Input: part model. Units: mm. Frame: model coordinates. Face numbers are marked on the shaded views. A direction names the side the tool comes from. Give positions to 0.01 mm unless a question says otherwise; leave off trailing zeros. Loops run counter-clockwise (first coordinate to the right, second up) from the corner with the lowest first, then second, coordinate; pieces in that order, holes last. Notation, with made-up numbers: (76, 76) -> (88, 76) arc R19 cw to (88, 106) -> close; hole circle Ø3 at (89, 17.25). An arc over 180 degrees is marked (long way). Answer as a JSON object with one key per item and string values.
```python
from build123d import *

# Parameters (mm, degrees)
F1_ANGLE_BACK = 135
F1_ANGLE      = 270
F3_DEPTH      = 29
F4_DEPTH      = 29


with BuildPart() as f1:
    # F0 (on Front) → F1 (revolve)
    with BuildSketch(Plane.XZ, mode=Mode.PRIVATE) as f1_sk:
        Polygon((0, -4), (0, 4), (-35, 4), (-35, 29), (-43, 29), (-43, -29), (-35, -29), (-35, -4), align=None)
    revolve(f1_sk.sketch.rotate(Axis((0, 0, -1.0322406888), (0, 0, 1)), -F1_ANGLE_BACK), axis=Axis((0, 0, -1.0322406888), (0, 0, 1)), revolution_arc=F1_ANGLE)

    # F2 (on Top) → F3 (join, through all)
    with BuildSketch(Plane.XY):
        Polygon((0, 0), (30.405591591, -30.405591591), (33.941125497, -26.8700576851), (7.0710678119, 0), (33.941125497, 26.8700576851), (30.405591591, 30.405591591), align=None)
    extrude(amount=F3_DEPTH)

    # F4 (add, through all): a face of the model
    f4_faces = [f1.faces().sort_by_distance(p)[0] for p in [
        (15.6952386856, -14.7103529054, 0),
    ]]
    extrude(f4_faces, amount=F4_DEPTH)


solid = f1.part
```
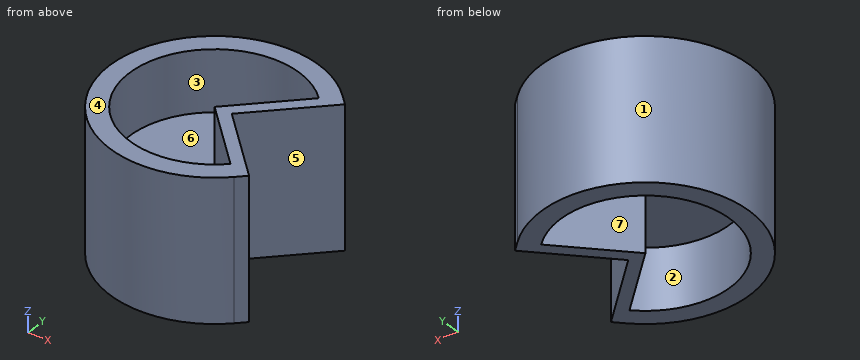
Q1. Section D-D, the plane x = 4. Return the cut outline in (y, z), then the cut area to 3 significant figures.
Evaluation:
{"outline": "(-42.81, -29) -> (-34.77, -29) -> (-34.77, -4) -> (-4, -4) -> (-4, -29) -> (4, -29) -> (4, -4) -> (34.77, -4) -> (34.77, -29) -> (42.81, -29) -> (42.81, 29) -> (34.77, 29) -> (34.77, 4) -> (4, 4) -> (4, 29) -> (-4, 29) -> (-4, 4) -> (-34.77, 4) -> (-34.77, 29) -> (-42.81, 29) -> close", "area": "1,890 mm2"}
Q2. Ray query, line 1 along X through (y, z) = (0, 10); line 2 along Y through (x, z) = (11, 21.5); line 3 along Y through (x, z) = (3.5, -10). Return the intervals inside material, ascending.
Evaluation:
{"line 1": "x = -43 to -35, 0 to 7.07", "line 2": "y = -41.57 to -33.23, -11 to -3.93, 3.93 to 11, 33.23 to 41.57", "line 3": "y = -42.86 to -34.82, -3.5 to 3.5, 34.82 to 42.86"}
Q3. Pin query (flat end, axial travel): pin 1 (1 mm diameter, centred on x = 0, y = -17.5, fed in from -Z); pin 2 (10 mm diameter, centred on x = -25, z = -15, fed in from +Y); pin 3 (18 mm diameter, centred on x = -19.5, y = 15.5, fed in from +Z). Return the tip coordinate at first contact, or that it passes through.
Evaluation:
{"pin 1": "stops at z = -4", "pin 2": "stops at y = 38.07", "pin 3": "stops at z = 4"}
Q4. Draft query along Y for the marked faces 1, 2, 3 and 4. Return one class per face: +Y half, -Y half, draft (parallel to the pull), parting line (faces both ways), or undercut.
Evaluation:
{"face 1": "parting line", "face 2": "undercut", "face 3": "undercut", "face 4": "draft"}
Q5. Section A-A, the plane x = 12. Return the cut outline in (y, z), then the cut area to 3 significant figures.
Evaluation:
{"outline": "(-41.29, -29) -> (-32.88, -29) -> (-32.88, -4) -> (-12, -4) -> (-12, -29) -> (-4.93, -29) -> (-4.93, 29) -> (-12, 29) -> (-12, 4) -> (-32.88, 4) -> (-32.88, 29) -> (-41.29, 29) -> close; (4.93, -29) -> (12, -29) -> (12, -4) -> (32.88, -4) -> (32.88, -29) -> (41.29, -29) -> (41.29, 29) -> (32.88, 29) -> (32.88, 4) -> (12, 4) -> (12, 29) -> (4.93, 29) -> close", "area": "2,130 mm2"}
Q6. Section B-B, the plane z = 9.5. Return the cut outline in (x, y).
Evaluation:
{"outline": "(7.07, 0) -> (33.94, 26.87) -> (30.41, 30.41) arc R43 ccw (long way) to (30.41, -30.41) -> (33.94, -26.87) -> close; hole (0, 0) -> (24.75, 24.75) arc R35 ccw (long way) to (24.75, -24.75) -> close"}
Q7. Access query for the marked faces 5, 6 and 7. Directions: +Z, -Z, +X, -X, +Y, -Y. A direction counts if a zero-diameter tool reaches every point of the face in a straight line with its end or side. Return the directions, or none.
Evaluation:
{"face 5": "+Z, -Z, +X", "face 6": "+Z", "face 7": "-Z"}
Q8. Section C-C, the plane y = 21.5. Return the cut outline in (x, z), then the cut area to 3 significant figures.
Evaluation:
{"outline": "(-37.24, -29) -> (-27.62, -29) -> (-27.62, -4) -> (21.5, -4) -> (21.5, -29) -> (28.57, -29) -> (28.57, 29) -> (21.5, 29) -> (21.5, 4) -> (-27.62, 4) -> (-27.62, 29) -> (-37.24, 29) -> close", "area": "1,360 mm2"}
